CAD build for the part. Positions are in the model's coordinates, mm. Coordinates: 2 decimals unless noted, no trailing zeros. Write each loop counter-clockwise with the first axis right and the second up, starting at its lowest first coordinate (ties: lowest second). Pieces come first, ordered by that corner, then holes.
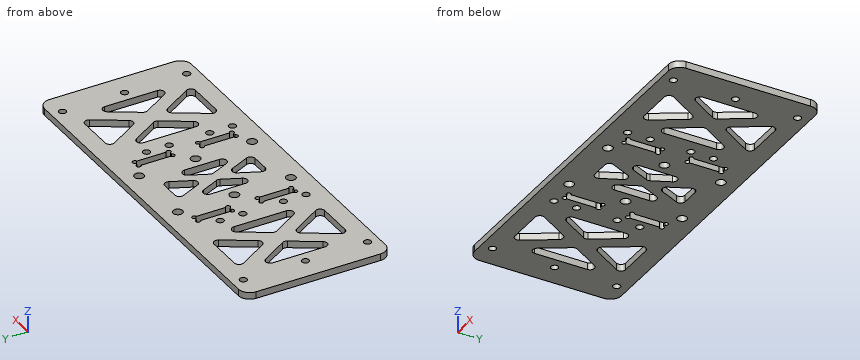
```python
from build123d import *

# Parameters (mm, degrees)
SKETCH_1_W          = 160
SKETCH_1_H          = 65
EXTRUDE_1_DEPTH     = 3
SKETCH_2_R          = 1.6
CUT_EXTRUDE_1_DEPTH = 173.725215299
SKETCH_3_R          = 2.1
CUT_EXTRUDE_2_DEPTH = 173.725215299
SKETCH_4_W          = 3
SKETCH_4_H          = 15
CUT_EXTRUDE_3_DEPTH = 173.725215299
SKETCH_5_R          = 1
CUT_EXTRUDE_4_DEPTH = 173.725215299
FILLET_1_R          = 5
SKETCH_6_R          = 1.6
CUT_EXTRUDE_5_DEPTH = 10
SKETCH_7_W          = 30
SKETCH_7_H          = 49
CUT_EXTRUDE_6_DEPTH = 10
SKETCH_8_W          = 20
SKETCH_8_H          = 40
CUT_EXTRUDE_7_DEPTH = 10
EXTRUDE_2_DEPTH     = 3
FILLET_3_R          = 2
SKETCH_10_W         = 3.4
SKETCH_10_H         = 15.4
CUT_EXTRUDE_8_DEPTH = 173.725215299


with BuildPart() as part:
    # 草图1 → 凸台-拉伸1 (new body)
    with BuildSketch(Plane.XY):
        with Locations((80, 32.5)):
            Rectangle(SKETCH_1_W, SKETCH_1_H)
    extrude(amount=EXTRUDE_1_DEPTH)

    # 草图2 → 切除-拉伸1 (cut, through all)
    with BuildSketch(Plane.XY.offset(3)):
        with Locations((150, 60)):
            Circle(SKETCH_2_R)
        with Locations((150, 32.5)):
            Circle(SKETCH_2_R)
        with Locations((150, 5)):
            Circle(SKETCH_2_R)
        with Locations(Location((10, 5, 0), (0, 0, 180))):
            Circle(SKETCH_2_R)
        with Locations(Location((10, 32.5, 0), (0, 0, 180))):
            Circle(SKETCH_2_R)
        with Locations(Location((10, 60, 0), (0, 0, 180))):
            Circle(SKETCH_2_R)
    extrude(amount=-CUT_EXTRUDE_1_DEPTH, mode=Mode.SUBTRACT)

    # 草图3 → 切除-拉伸2 (cut, through all)
    with BuildSketch(Plane.XY.offset(3)):
        with Locations((65, 57.5)):
            Circle(SKETCH_3_R)
        with Locations((65, 32.5)):
            Circle(SKETCH_3_R)
        with Locations(Location((65, 7.5, 0), (0, 0, 180))):
            Circle(SKETCH_3_R)
        with Locations((95, 7.5)):
            Circle(SKETCH_3_R)
        with Locations(Location((95, 32.5, 0), (0, 0, 180))):
            Circle(SKETCH_3_R)
        with Locations(Location((95, 57.5, 0), (0, 0, 180))):
            Circle(SKETCH_3_R)
    extrude(amount=-CUT_EXTRUDE_2_DEPTH, mode=Mode.SUBTRACT)

    # 草图4 → 切除-拉伸3 (cut, through all)
    with BuildSketch(Plane.XY.offset(3)):
        with Locations((57, 46.5)):
            Rectangle(SKETCH_4_W, SKETCH_4_H)
        with Locations((57, 18.5)):
            Rectangle(SKETCH_4_W, SKETCH_4_H)
        with Locations((103, 18.5)):
            Rectangle(SKETCH_4_W, SKETCH_4_H)
        with Locations((103, 46.5)):
            Rectangle(SKETCH_4_W, SKETCH_4_H)
    extrude(amount=-CUT_EXTRUDE_3_DEPTH, mode=Mode.SUBTRACT)

    # 草图5 → 切除-拉伸4 (cut, through all)
    with BuildSketch(Plane.XY.offset(3)):
        with Locations((58.5, 54)):
            Circle(SKETCH_5_R)
        with Locations((55.5, 54)):
            Circle(SKETCH_5_R)
        with Locations((58.5, 39)):
            Circle(SKETCH_5_R)
        with Locations((55.5, 39)):
            Circle(SKETCH_5_R)
        with Locations((58.5, 26)):
            Circle(SKETCH_5_R)
        with Locations((55.5, 26)):
            Circle(SKETCH_5_R)
        with Locations((58.5, 11)):
            Circle(SKETCH_5_R)
        with Locations((55.5, 11)):
            Circle(SKETCH_5_R)
        with Locations((104.5, 54)):
            Circle(SKETCH_5_R)
        with Locations((101.5, 54)):
            Circle(SKETCH_5_R)
        with Locations((104.5, 39)):
            Circle(SKETCH_5_R)
        with Locations((101.5, 39)):
            Circle(SKETCH_5_R)
        with Locations((104.5, 26)):
            Circle(SKETCH_5_R)
        with Locations((101.5, 26)):
            Circle(SKETCH_5_R)
        with Locations((104.5, 11)):
            Circle(SKETCH_5_R)
        with Locations((101.5, 11)):
            Circle(SKETCH_5_R)
    extrude(amount=-CUT_EXTRUDE_4_DEPTH, mode=Mode.SUBTRACT)

    # 圆角1
    fillet_1_edges = [part.edges().sort_by_distance(p)[0] for p in [
        (0, 65, 1.5),
        (160, 65, 1.5),
        (160, 0, 1.5),
        (0, 0, 1.5),
    ]]
    fillet(fillet_1_edges, radius=FILLET_1_R)

    # 草图6 → 切除-拉伸5 (cut)
    with BuildSketch(Plane.XY.offset(3)):
        with Locations((108.5, 46.5)):
            Circle(SKETCH_6_R)
        with Locations((108.5, 36.5)):
            Circle(SKETCH_6_R)
        with Locations((108.5, 18.5)):
            Circle(SKETCH_6_R)
        with Locations((108.5, 8.5)):
            Circle(SKETCH_6_R)
        with Locations(Location((51.5, 8.5, 0), (0, 0, 180))):
            Circle(SKETCH_6_R)
        with Locations(Location((51.5, 18.5, 0), (0, 0, 180))):
            Circle(SKETCH_6_R)
        with Locations(Location((51.5, 36.5, 0), (0, 0, 180))):
            Circle(SKETCH_6_R)
        with Locations(Location((51.5, 46.5, 0), (0, 0, 180))):
            Circle(SKETCH_6_R)
    extrude(amount=-CUT_EXTRUDE_5_DEPTH, mode=Mode.SUBTRACT)

    # 草图7 → 切除-拉伸6 (cut)
    with BuildSketch(Plane.XY.offset(3)):
        with Locations((130, 32.5)):
            Rectangle(SKETCH_7_W, SKETCH_7_H)
        with Locations((30, 32.5)):
            Rectangle(SKETCH_7_W, SKETCH_7_H)
    extrude(amount=-CUT_EXTRUDE_6_DEPTH, mode=Mode.SUBTRACT)

    # 草图8 → 切除-拉伸7 (cut)
    with BuildSketch(Plane.XY.offset(3)):
        with Locations((80, 32.5)):
            Rectangle(SKETCH_8_W, SKETCH_8_H)
    extrude(amount=-CUT_EXTRUDE_7_DEPTH, mode=Mode.SUBTRACT)

    # 草图9 → 凸台-拉伸2 (add, through all)
    with BuildSketch(Plane.XY.offset(3)):
        Polygon((45, 13.745432969), (45, 8), (41.482387978, 8), (30, 26.754567031), (18.517612022, 8), (15, 8), (15, 13.745432969), (26.482387978, 32.5), (15, 51.254567031), (15, 57), (18.517612022, 57), (30, 38.245432969), (41.482387978, 57), (45, 57), (45, 51.254567031), (33.517612022, 32.5), align=None)
        Polygon((82.201517486, 32.5), (90, 15.549573016), (90, 12.5), (87, 12.5), (80, 27.714881699), (73, 12.5), (70, 12.5), (70, 15.549573016), (77.798482514, 32.5), (70, 49.450426984), (70, 52.5), (73, 52.5), (80, 37.285118301), (87, 52.5), (90, 52.5), (90, 49.450426984), align=None)
        Polygon((130, 26.754567031), (118.517612022, 8), (115, 8), (115, 13.745432969), (126.482387978, 32.5), (115, 51.254567031), (115, 57), (118.517612022, 57), (130, 38.245432969), (141.482387978, 57), (145, 57), (145, 51.254567031), (133.517612022, 32.5), (145, 13.745432969), (145, 8), (141.482387978, 8), align=None)
    extrude(amount=-EXTRUDE_2_DEPTH)

    # 圆角3
    fillet_3_edges = [part.edges().sort_by_distance(p)[0] for p in [
        (45, 13.745432969, 1.5),
        (41.482387978, 8, 1.5),
        (30, 26.754567031, 1.5),
        (18.517612022, 8, 1.5),
        (15, 13.745432969, 1.5),
        (26.482387978, 32.5, 1.5),
        (15, 51.254567031, 1.5),
        (18.517612022, 57, 1.5),
        (30, 38.245432969, 1.5),
        (41.482387978, 57, 1.5),
        (45, 51.254567031, 1.5),
        (33.517612022, 32.5, 1.5),
        (82.201517486, 32.5, 1.5),
        (90, 15.549573016, 1.5),
        (87, 12.5, 1.5),
        (80, 27.714881699, 1.5),
        (73, 12.5, 1.5),
        (70, 15.549573016, 1.5),
        (77.798482514, 32.5, 1.5),
        (70, 49.450426984, 1.5),
        (73, 52.5, 1.5),
        (80, 37.285118301, 1.5),
        (87, 52.5, 1.5),
        (90, 49.450426984, 1.5),
        (130, 26.754567031, 1.5),
        (118.517612022, 8, 1.5),
        (115, 13.745432969, 1.5),
        (126.482387978, 32.5, 1.5),
        (115, 51.254567031, 1.5),
        (118.517612022, 57, 1.5),
        (130, 38.245432969, 1.5),
        (141.482387978, 57, 1.5),
        (145, 51.254567031, 1.5),
        (133.517612022, 32.5, 1.5),
        (145, 13.745432969, 1.5),
        (141.482387978, 8, 1.5),
    ]]
    fillet(fillet_3_edges, radius=FILLET_3_R)

    # 草图10 → 切除-拉伸8 (cut, through all)
    with BuildSketch(Plane.XY.offset(3)):
        with Locations((103, 46.5)):
            Rectangle(SKETCH_10_W, SKETCH_10_H)
        with Locations((103, 18.5)):
            Rectangle(SKETCH_10_W, SKETCH_10_H)
        with Locations((57, 18.5)):
            Rectangle(SKETCH_10_W, SKETCH_10_H)
        with Locations((57, 46.5)):
            Rectangle(SKETCH_10_W, SKETCH_10_H)
    extrude(amount=-CUT_EXTRUDE_8_DEPTH, mode=Mode.SUBTRACT)


solid = part.part
```
Item 1: Saw through at B-B, the plane z = 0.5. State how many separate pieces and enclosed holes the cut face has, and give its area (3 significant figures).
Item 2: Wall check: line 1 along Y through (x, z) = (108.5, 2.05); line 2 along Y through (x, z) = (129, 0.35); line 3 along Y through (x, z) = (58.5, 2.4). Give the ranges that are in metal, low to high.
Item 3: Saw through at A-A, the plane y = 28.5. Write the cut outline in (x, z), and give its area (3 significant figures).
Working result:
1. separate pieces: 1
1. enclosed holes: 36
1. area: 7,920 mm2
2. line 1: y = 0 to 6.9, 10.1 to 16.9, 20.1 to 34.9, 38.1 to 44.9, 48.1 to 65
2. line 2: y = 0 to 8, 24.66 to 40.34, 57 to 65
2. line 3: y = 0 to 10, 27 to 38, 55 to 65
3. outline: (0, 0) - (15, 0) - (15, 3) - (0, 3) - close; (24.03, 0) - (35.97, 0) - (35.97, 3) - (24.03, 3) - close; (45, 0) - (70, 0) - (70, 3) - (45, 3) - close; (75.96, 0) - (84.04, 0) - (84.04, 3) - (75.96, 3) - close; (90, 0) - (115, 0) - (115, 3) - (90, 3) - close; (124.03, 0) - (135.97, 0) - (135.97, 3) - (124.03, 3) - close; (145, 0) - (160, 0) - (160, 3) - (145, 3) - close
3. area: 336 mm2
